from build123d import *

# Parameters (mm, degrees)
F0_R     = 3.9624
F0_R_2   = 5.1562
F1_DEPTH = 31.6992
F0_R_3   = 8.7376
F2_DEPTH = 9.4742
F4_DEPTH = 19.05


with BuildPart() as f1:
    # F0 (on Front) → F1 (new body)
    with BuildSketch(Plane.XZ):
        with BuildLine():
            ThreePointArc((-53.9418684482, 1.8908869118), (-0.945588575, -53.9667164764), (53.975, 0))
            ThreePointArc((53.975, 0), (14.14638739, 52.0881977881), (-46.559704912, 27.3037452286))
            Line((-46.559704912, 27.3037452286), (-24.1670829241, 11.1631898628))
            ThreePointArc((-24.1670829241, 11.1631898628), (-3.9962450465, 44.3324916596), (25.4631440543, 19.0498953495))
            ThreePointArc((25.4631440543, 19.0498953495), (44.449999882, -0.0021200322), (25.4589040116, -19.049908932))
            ThreePointArc((25.4589040116, -19.049908932), (0.2533724347, -44.9959238654), (-25.463489659, -19.5566330526))
            Line((-25.463489659, -19.5566330526), (-53.9418684482, 1.8908869118))
        make_face()
        with Locations((-31.9465398788, -31.6641107202)):
            Circle(F0_R, mode=Mode.SUBTRACT)
        with Locations((31.6804601212, -31.6641107202)):
            Circle(F0_R_2, mode=Mode.SUBTRACT)
        with Locations((-31.9465398788, 31.9628892798)):
            Circle(F0_R, mode=Mode.SUBTRACT)
        with Locations((31.6804601212, 31.9628892798)):
            Circle(F0_R_2, mode=Mode.SUBTRACT)
        with BuildLine():
            Line((-24.1670829241, 11.1631898628), (-46.559704912, 27.3037452286))
            ThreePointArc((-46.559704912, 27.3037452286), (-51.8323731265, 15.0567500169), (-53.9418684482, 1.8908869118))
            Line((-53.9418684482, 1.8908869118), (-25.463489659, -19.5566330526))
            ThreePointArc((-25.463489659, -19.5566330526), (-23.1304283544, -8.8860032088), (-16.5413044773, -0.174576067))
            ThreePointArc((-16.5413044773, -0.174576067), (-21.1288768106, 4.9732552376), (-24.1670829241, 11.1631898628))
        make_face()
    extrude(amount=F1_DEPTH)

    # F0 (on Front) → F2 (join)
    with BuildSketch(Plane.XZ):
        with BuildLine():
            ThreePointArc((25.4631440543, 19.0498953495), (-3.9962450465, 44.3324916596), (-24.1670829241, 11.1631898628))
            ThreePointArc((-24.1670829241, 11.1631898628), (-21.1288768106, 4.9732552376), (-16.5413044773, -0.174576067))
            ThreePointArc((-16.5413044773, -0.174576067), (-23.1304283544, -8.8860032088), (-25.463489659, -19.5566330526))
            ThreePointArc((-25.463489659, -19.5566330526), (0.2533724347, -44.9959238654), (25.4589040116, -19.049908932))
            ThreePointArc((25.4589040116, -19.049908932), (23.0233343799, -8.6563729399), (16.5413044773, -0.174576067))
            ThreePointArc((16.5413044773, -0.174576067), (23.0973699676, 8.4653284163), (25.4631440543, 19.0498953495))
        make_face()
        with Locations((0, -19.5336844772)):
            Circle(F0_R_3, mode=Mode.SUBTRACT)
        with Locations((0, 19.1845323432)):
            Circle(F0_R_3, mode=Mode.SUBTRACT)
        with BuildLine():
            ThreePointArc((25.4589040116, -19.049908932), (44.449999882, -0.0021200322), (25.4631440543, 19.0498953495))
            ThreePointArc((25.4631440543, 19.0498953495), (23.0973699676, 8.4653284163), (16.5413044773, -0.174576067))
            ThreePointArc((16.5413044773, -0.174576067), (23.0233343799, -8.6563729399), (25.4589040116, -19.049908932))
        make_face()
    extrude(amount=F2_DEPTH)

    # F3 (on face) → F4 (cut)
    with BuildSketch(Plane.XZ.offset(31.6992)):
        with BuildLine():
            ThreePointArc((-16.5413044773, -0.174576067), (-22.6355522481, 7.5217022119), (-25.3653949946, 16.9514696437))
            Line((-25.3653949946, 16.9514696437), (-43.0676051814, 32.5343204776))
            ThreePointArc((-43.0676051814, 32.5343204776), (-50.3270192168, 19.5061980343), (-53.7439555951, 4.988773596))
            Line((-53.7439555951, 4.988773596), (-25.4202754774, -21.0167309709))
            ThreePointArc((-25.4202754774, -21.0167309709), (-23.4263186039, -9.5538333302), (-16.5413044773, -0.174576067))
        make_face()
    extrude(amount=-F4_DEPTH, mode=Mode.SUBTRACT)


solid = f1.part
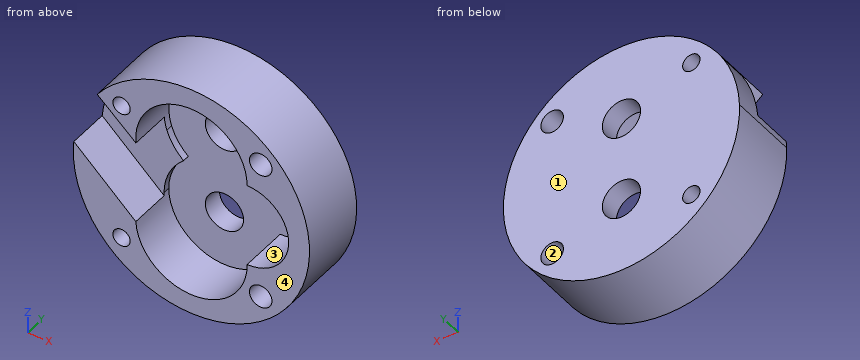
Source: CAD feature listing. Evaluate the final solid. Frame: model axes, mm. Face numbers are marked on the shaded views. A direction names the side the tool comes from. Round coordinates to 2 decimals unless told otherwise and drop trailing zeros. Loops run counter-clockwise (first coordinate to the right, second up) from the corner with the lowest first, then second, coordinate; pieces in that order, holes last. Notation, with made-up numbers: (-28, -6) - (-19, -6) arc R18 ccw to (-19, 23) - close; hole circle Ø1 at (-25.75, 71.25). An arc over 180 degrees is marked (long way). Write item = value, one per line. Start each with the question number.
(1) Ray query, line 1 along Z through (x, y) = (0, -4) (3 decimals); line 2 along X through (y, z) = (-27.5, -30); line 3 along Y through (x, z) = (-17, -19.5). Return the intervals inside material, ascending. Write a range as from..to.
(2) Set-up query: the marked faces 3 and 4. Return all of +Z, -Z, +X, -X, +Y, -Y with unobstructed straight access to the full face (end or side cutting, diameter ignored); none if empty.
(3) Section query A-A, the plane x = 0. Output: boundary loops of the cut face in (y, z) (3 decimals), plus the area to 3 significant figures.
(4) Section query B-B, the plane z = -33.5. Output: boundary loops of the cut face in (x, y), plus the area to 3 significant figures.
(5) Pin query (flat end, axial travel): pin 1 (22.5 mm diameter, centred on x = 0, z = -19.53, fed in from -Y); pin 2 (10 mm diameter, centred on x = -1, y = -3.5, fed in from +Z) (3 decimals); pin 3 (2 mm diameter, centred on x = 9, y = -12, fed in from +Z); pin 4 (5 mm diameter, centred on x = -31.95, z = -31.66, fed in from -Y). Return the tip coordinate at first contact, or that it passes through.
(6) Pull-direction query (X, two-part tool) for the marked faces 1 and 2; classes: +X half, -X half, draft (parallel to the pull), parting line (faces both ways), or undercut.
(7) Section query D-D, the plane x = 16.5. Output: boundary loops of the cut face in (y, z).
(8) Section query C-C, the plane y = -19.5. State how many separate pieces and enclosed holes the cut face has, plus the area to 3 significant figures.
Conclusion:
q1.line_1 = -53.975..-28.271, -10.796..10.447, 27.922..53.975
q1.line_2 = -44.87..-35.54, -28.35..-23.21, 23.21..26.8, 36.56..44.87
q1.line_3 = -9.47..0
q2.face_3 = -Y
q2.face_4 = +Z, -Z, +X, -X, -Y
q3.outline = (-31.699, -53.975) - (0, -53.975) - (0, -28.271) - (-9.474, -28.271) - (-9.474, -44.997) - (-31.699, -44.997) - close; (-31.699, 44.648) - (-9.474, 44.648) - (-9.474, 27.922) - (0, 27.922) - (0, 53.975) - (-31.699, 53.975) - close; (-9.474, -10.796) - (0, -10.796) - (0, 10.447) - (-9.474, 10.447) - close
q3.area = 1,100 mm2
q4.outline = (-42.32, -31.7) - (-35.46, -31.7) - (-35.46, 0) - (-42.32, 0) - close; (-28.44, -31.7) - (-21.29, -31.7) - (-21.29, -9.47) - (21.29, -9.47) - (21.29, -31.7) - (26.86, -31.7) - (26.86, 0) - (-28.44, 0) - close; (36.5, -31.7) - (42.32, -31.7) - (42.32, 0) - (36.5, 0) - close
q4.area = 1,210 mm2
q5.pin_1 = -9.47
q5.pin_2 = 53.975
q5.pin_3 = 53.38
q5.pin_4 = through
q6.face_1 = draft
q6.face_2 = undercut
q7.outline = (-31.7, -51.39) - (0, -51.39) - (0, 51.39) - (-31.7, 51.39) - (-31.7, 38.58) - (-9.47, 38.58) - (-9.47, -38.93) - (-31.7, -38.93) - close
q8.separate_pieces = 1
q8.enclosed_holes = 4
q8.area = 3,410 mm2
